from build123d import *
from build123d.topology import SkipClean

# Parameters (mm, degrees)
BOSS_EXTRUDE1_DEPTH     = 165.1
SKETCH2_R               = 88.9
BOSS_EXTRUDE2_DEPTH     = 228.6
SKETCH3_R               = 127
BOSS_EXTRUDE3_DEPTH     = 12.7
SKETCH4_W               = 152.4
SKETCH4_H               = 152.4
BOSS_EXTRUDE4_DEPTH     = 209.55
SKETCH5_W               = 25.4
SKETCH5_H               = 11.43
CUT_EXTRUDE1_DEPTH      = 209.55
LPATTERN1_COUNT         = 4
LPATTERN1_PITCH         = 22.86
MIRROR1_COPY_1_SKETCH_W = 25.4
MIRROR1_COPY_1_SKETCH_H = 11.43
MIRROR1_COPY_1_DEPTH    = 209.55
MIRROR1_COPY_2_SKETCH_W = 25.4
MIRROR1_COPY_2_SKETCH_H = 11.43
MIRROR1_COPY_2_DEPTH    = 209.55
MIRROR1_COPY_3_SKETCH_W = 25.4
MIRROR1_COPY_3_SKETCH_H = 11.43
MIRROR1_COPY_3_DEPTH    = 209.55
SKETCH7_R               = 76.2
CUT_EXTRUDE2_DEPTH      = 228.6
SKETCH8_R               = 19.05
CUT_EXTRUDE3_DEPTH      = 228.6
SKETCH9_R               = 9.525
CUT_EXTRUDE5_DEPTH      = 50.8


with BuildPart() as part:
    # Sketch1 → Boss-Extrude1 (new body)
    with BuildSketch(Plane(origin=(0, 0, 0), x_dir=(0, 0, -1), z_dir=(1, 0, 0))):
        with BuildLine():
            Line((-152.4, -171.45), (152.4, -171.45))
            Line((152.4, -171.45), (84.14126771, 28.695941668))
            ThreePointArc((84.14126771, 28.695941668), (0, 88.9), (-84.14126771, 28.695941668))
            Line((-84.14126771, 28.695941668), (-152.4, -171.45))
        make_face()
    extrude(amount=BOSS_EXTRUDE1_DEPTH)

    # Sketch2 → Boss-Extrude2 (add)
    with SkipClean():  # the faces are left unmerged after this step: merging them gives an invalid solid
        with BuildSketch(Plane.ZY):
            Circle(SKETCH2_R)
        extrude(amount=-BOSS_EXTRUDE2_DEPTH)

    # Sketch3 → Boss-Extrude3 (add)
    with BuildSketch(Plane(origin=(228.6, 0, 0), x_dir=(0, 0, -1), z_dir=(1, 0, 0))):
        Circle(SKETCH3_R)
    extrude(amount=BOSS_EXTRUDE3_DEPTH)

    # Sketch4 → Boss-Extrude4 (add)
    with BuildSketch(Plane.ZY.offset(-228.6)):
        with Locations((0, 76.2)):
            Rectangle(SKETCH4_W, SKETCH4_H)
    extrude(amount=BOSS_EXTRUDE4_DEPTH)

    # Sketch5 → Cut-Extrude1 (cut)
    with BuildSketch(Plane.ZY.offset(-19.05)):
        with Locations((-76.2, 135.255)):
            Rectangle(SKETCH5_W, SKETCH5_H)
    cut_extrude1 = extrude(amount=-CUT_EXTRUDE1_DEPTH, mode=Mode.SUBTRACT)

    # LPattern1: Cut-Extrude1 ×4
    with Locations(*[(0, -i * LPATTERN1_PITCH, 0) for i in range(1, LPATTERN1_COUNT)]):
        add(cut_extrude1, mode=Mode.SUBTRACT)

    # Mirror1: Cut-Extrude1 across plane
    add(cut_extrude1.mirror(Plane.XY), mode=Mode.SUBTRACT)

    # Mirror1 copy 1 sketch → Mirror1 copy 1 (cut)
    with BuildSketch(Plane(origin=(19.05, -22.86, 0), x_dir=(0, 0, -1), z_dir=(-1, 0, 0))):
        with Locations((-76.2, -135.255)):
            Rectangle(MIRROR1_COPY_1_SKETCH_W, MIRROR1_COPY_1_SKETCH_H)
    extrude(amount=-MIRROR1_COPY_1_DEPTH, mode=Mode.SUBTRACT)

    # Mirror1 copy 2 sketch → Mirror1 copy 2 (cut)
    with BuildSketch(Plane(origin=(19.05, -45.72, 0), x_dir=(0, 0, -1), z_dir=(-1, 0, 0))):
        with Locations((-76.2, -135.255)):
            Rectangle(MIRROR1_COPY_2_SKETCH_W, MIRROR1_COPY_2_SKETCH_H)
    extrude(amount=-MIRROR1_COPY_2_DEPTH, mode=Mode.SUBTRACT)

    # Mirror1 copy 3 sketch → Mirror1 copy 3 (cut)
    with BuildSketch(Plane(origin=(19.05, -68.58, 0), x_dir=(0, 0, -1), z_dir=(-1, 0, 0))):
        with Locations((-76.2, -135.255)):
            Rectangle(MIRROR1_COPY_3_SKETCH_W, MIRROR1_COPY_3_SKETCH_H)
    extrude(amount=-MIRROR1_COPY_3_DEPTH, mode=Mode.SUBTRACT)

    # Sketch7 → Cut-Extrude2 (cut)
    with BuildSketch(Plane(origin=(241.3, 0, 0), x_dir=(0, 0, -1), z_dir=(1, 0, 0))):
        Circle(SKETCH7_R)
    extrude(amount=-CUT_EXTRUDE2_DEPTH, mode=Mode.SUBTRACT)

    # Sketch8 → Cut-Extrude3 (cut)
    with BuildSketch(Plane(origin=(12.7, 0, 0), x_dir=(0, 0, -1), z_dir=(1, 0, 0))):
        Circle(SKETCH8_R)
    extrude(amount=-CUT_EXTRUDE3_DEPTH, mode=Mode.SUBTRACT)

    # Sketch9 → Cut-Extrude5 (cut)
    with BuildSketch(Plane(origin=(241.3, 0, 0), x_dir=(0, 0, -1), z_dir=(1, 0, 0))):
        with Locations((0, -107.95)):
            Circle(SKETCH9_R)
        with Locations((-93.487442339, 53.975)):
            Circle(SKETCH9_R)
        with Locations((93.487442339, 53.975)):
            Circle(SKETCH9_R)
    extrude(amount=-CUT_EXTRUDE5_DEPTH, mode=Mode.SUBTRACT)


solid = part.part
Verification items for the finished model (mm, model axes). A direction names the side the tool comes from. Give positions to 0.01 mm unless a question says otherwise; leave off trailing zeros. Loops run counter-clockwise (first coordinate to the right, second up) from the corner with the lowest first, then second, coordinate; pieces in that order, holes last.
1) Set-up check for faces 1 (the flat face through (122, 135, 63.5)), 2 (the flat face through (122, 83.82, -70)), 3 (the flat face through (125, 147, 76.2)), 4 (the flat face through (122, 135, -63.5)): record each of +Z, -Z, +X, -X, +Y, -Y from which the full face is reachable in a straight line by a thin tool's end or side.
2) Thickness scan on line 1 along Y through (x, z) = (9, 0); line 2 along X through (y, z) = (-96, 8.5); line 3 along Y through (x, z) = (34, -3). Record the ranges inside material, lowest first.
3) Sectioned sample at C-C, the plane y = 0. Enter the section's corners in (x, z), then the cut area to 3 significant figures.
4) Sectioned sample at D-D, the plane z = -39.5. Enter the section's corners in (x, y).
5) Draft check along Y on faces 5 (the flat face through (122, 60.96, 70)), 6 (the flat face through (122, 95.25, 70)), 7 (the flat face through (241.3, -55, -55)), 8 (the cylindrical face through (234.86, -123.98, 27.53)). Enter one of: pulls with the +Y half, pulls with the -Y half, needs draft (parallel to the pull), parting line crosses it, or undercut.
6) Sectioned sample at B-B, the plane y = -107.95. Enter the section's corners in (x, z) (3 decimals), then the cut area to 3 significant figures.
7) Depth check by flat-ended pin: pin 1 Ø12.5 at (x, y) = (115.5, 67.5) entering from +Z; pin 2 Ø10 at (y, z) = (-92.5, -23) entering from -X; pin 3 Ø4 at (x, z) = (204.5, -16.5) entering from -Y; pin 4 Ø10 at (y, z) = (-24, 45) entering from +X. Enter the tip coordinate at first touch or a pass-through.
8) Sectioned sample at A-A, the plane z = 0. Enter the section's corners in (x, y) (3 decimals).
Answers:
1. face 1: +Z, +X, -X
1. face 2: -Z, -X
1. face 3: +Z, +X, -X, +Y
1. face 4: -Z, +X, -X
2. line 1: y = -171.45 to -19.05, 19.05 to 88.9
2. line 2: x = 0 to 165.1, 228.6 to 241.3
2. line 3: y = -171.45 to -76.14, 76.14 to 152.4
3. outline: (0, -93.93) - (165.1, -93.93) - (165.1, -88.9) - (228.6, -88.9) - (228.6, -127) - (241.3, -127) - (241.3, -76.2) - (12.7, -76.2) - (12.7, -19.05) - (0, -19.05) - close; (0, 19.05) - (12.7, 19.05) - (12.7, 76.2) - (241.3, 76.2) - (241.3, 127) - (228.6, 127) - (228.6, 88.9) - (165.1, 88.9) - (165.1, 93.93) - (0, 93.93) - close
3. area: 10,200 mm2
4. outline: (0, -171.45) - (165.1, -171.45) - (165.1, -79.64) - (228.6, -79.64) - (228.6, -120.7) - (241.3, -120.7) - (241.3, -65.16) - (12.7, -65.16) - (12.7, 65.16) - (241.3, 65.16) - (241.3, 120.7) - (228.6, 120.7) - (228.6, 152.4) - (19.05, 152.4) - (19.05, 79.64) - (0, 79.64) - close
5. face 5: undercut
5. face 6: undercut
5. face 7: needs draft
5. face 8: parting line crosses it
6. outline: (0, -130.744) - (165.1, -130.744) - (165.1, 130.744) - (0, 130.744) - close; (228.6, -66.901) - (241.3, -66.901) - (241.3, -9.525) - (228.6, -9.525) - close; (228.6, 9.525) - (241.3, 9.525) - (241.3, 66.901) - (228.6, 66.901) - close
6. area: 44,600 mm2
7. pin 1: stops at z = 76.2
7. pin 2: stops at x = 0
7. pin 3: stops at y = -87.71
7. pin 4: stops at x = 12.7
8. outline: (0, -171.45) - (165.1, -171.45) - (165.1, -88.9) - (228.6, -88.9) - (228.6, -98.425) - (241.3, -98.425) - (241.3, -76.2) - (12.7, -76.2) - (12.7, -19.05) - (0, -19.05) - close; (0, 19.05) - (12.7, 19.05) - (12.7, 76.2) - (241.3, 76.2) - (241.3, 127) - (228.6, 127) - (228.6, 152.4) - (19.05, 152.4) - (19.05, 88.9) - (0, 88.9) - close; (228.6, -127) - (241.3, -127) - (241.3, -117.475) - (228.6, -117.475) - close
